The drawing under review shows one solid part. Ordinate dimensions are in mm from its lowest x, y, z. Coordinates: 2 decimals unless noted, no trailing zeros. Order: outer loops, then holes, each group sorted by start corner. A loop starts at its lowest first (then second) coordinate and runs counter-clockwise, first axis right, second up. Notation, with made-up numbers: M -36,11 L -16,11 A12 cw -16,20 Z; hole C -31.5,35 d2. An arc over 180 degrees is marked long. Answer as a JSON object with one key per item and string values.
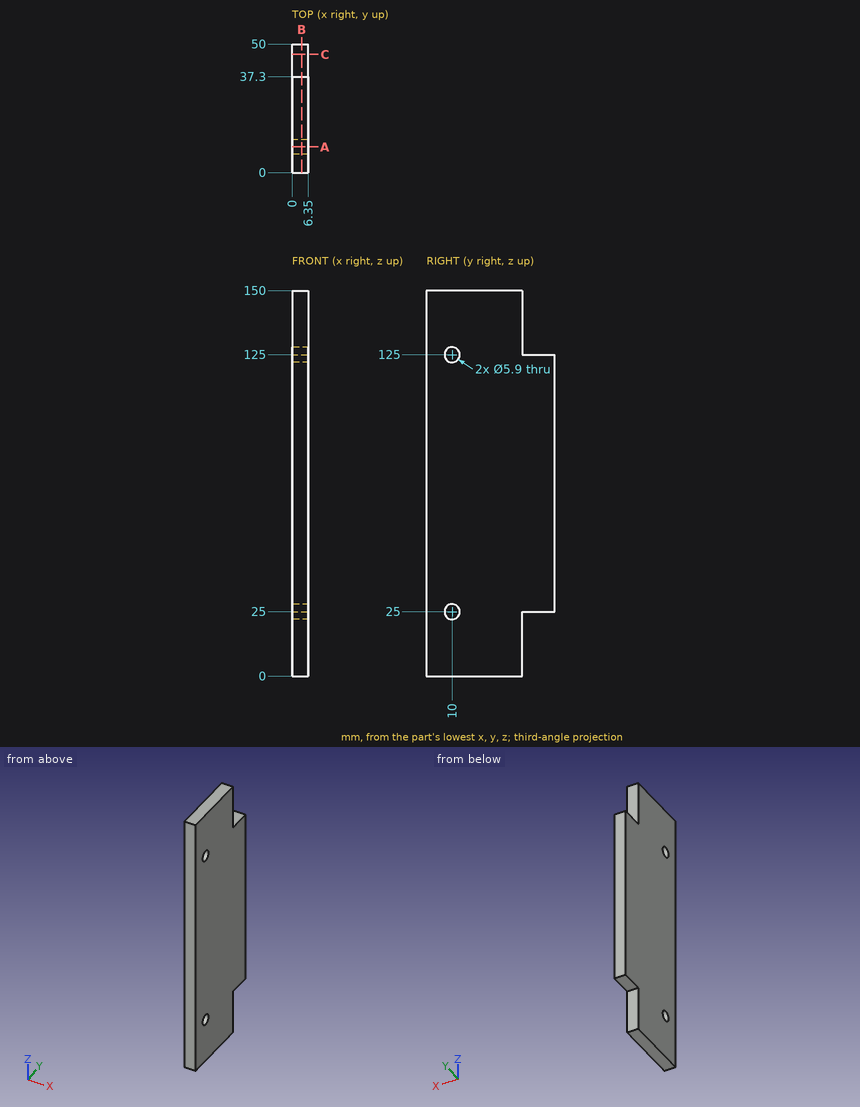
1) To check wall thickness, follow L1, parallel to Z at x = 4, y = 10; L2, parallel to Y at x = 3, z = 8.5; L3, parallel to Y at x = 1.5, z = 127. State the ranges of each line that lie inside material, in increasing order.
Taken from the geometry:
{"L1": "z = 0 to 22.05, 27.95 to 122.05, 127.95 to 150", "L2": "y = 0 to 37.3", "L3": "y = 0 to 7.83, 12.17 to 37.3"}
2) Add section A-A (y = 10). State the section outline as (x, z) points.
Taken from the geometry:
{"outline": "M 0,0 L 6.35,0 L 6.35,22.05 L 0,22.05 Z; M 0,27.95 L 6.35,27.95 L 6.35,122.05 L 0,122.05 Z; M 0,127.95 L 6.35,127.95 L 6.35,150 L 0,150 Z"}
3) Insertion check: pin 1 Ø3 at (x, z) = (3.5, 6.5) entering from +Y; pin 2 Ø1.9 at (x, y) = (3, 45.5) entering from -Z; pin 3 Ø5.5 at (y, z) = (10, 25) entering from +X; pin 4 Ø7.5 at (y, z) = (10, 125) entering from +X. Each pin has a flat end and moves straight along its axis. Give the tip position at first contact, or say it passes through.
Taken from the geometry:
{"pin 1": "stops at y = 37.3", "pin 2": "stops at z = 25", "pin 3": "passes through", "pin 4": "stops at x = 6.35"}
4) Add section C-C (y = 46). State the section outline as (x, z) points, and give its area (3 significant figures).
Taken from the geometry:
{"outline": "M 0,25 L 6.35,25 L 6.35,125 L 0,125 Z", "area": "635 mm2"}
5) Add section B-B (x = 3.75). State the section outline as (y, z) points.
Taken from the geometry:
{"outline": "M 0,0 L 37.3,0 L 37.3,25 L 50,25 L 50,125 L 37.3,125 L 37.3,150 L 0,150 Z; hole C 10,25 d5.9; hole C 10,125 d5.9"}
